```python
from build123d import *

# Parameters (mm, degrees)
SCHIZZO1_W                   = 75
SCHIZZO1_H                   = 60
ESTRUSIONE_ESTRUSIONE1_DEPTH = 5
SCHIZZO2_R                   = 5
TAGLIO_ESTRUSIONE1_DEPTH     = 49.28301979
SCHIZZO3_W                   = 45
SCHIZZO3_H                   = 5
ESTRUSIONE_ESTRUSIONE2_DEPTH = 8


with BuildPart() as part:
    # Schizzo1 → Estrusione-Estrusione1 (new body)
    with BuildSketch(Plane(origin=(0, 0, 0), x_dir=(1, 0, 0), z_dir=(0, 1, 0))):
        Rectangle(SCHIZZO1_W, SCHIZZO1_H)
    extrude(amount=ESTRUSIONE_ESTRUSIONE1_DEPTH)

    # Schizzo2 → Taglio-Estrusione1 (cut, through all)
    with BuildSketch(Plane(origin=(0, 5, 0), x_dir=(-1, 0, 0), z_dir=(0, 1, 0))):
        with Locations(Location((0, 0, 0), (0, 0, 90))):
            Circle(SCHIZZO2_R)
    extrude(amount=-TAGLIO_ESTRUSIONE1_DEPTH, mode=Mode.SUBTRACT)

    # Schizzo3 → Estrusione-Estrusione2 (add)
    with BuildSketch(Plane.XY.offset(30)):
        with Locations((0, 2.5)):
            Rectangle(SCHIZZO3_W, SCHIZZO3_H)
    estrusione_estrusione2 = extrude(amount=ESTRUSIONE_ESTRUSIONE2_DEPTH)

    # Specchia1: Estrusione-Estrusione2 across plane
    add(estrusione_estrusione2.mirror(Plane.XY))


solid = part.part
```
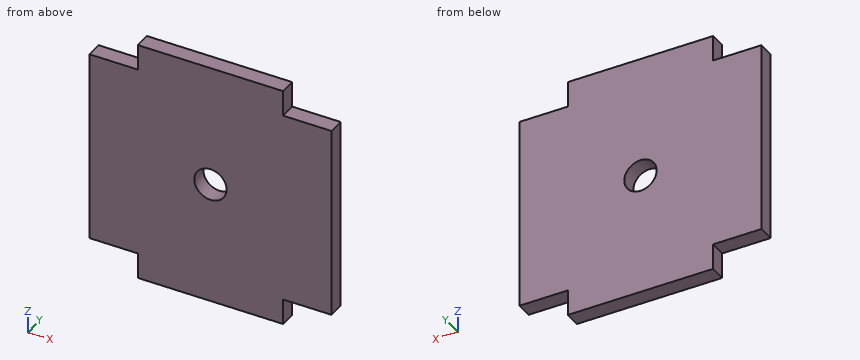
Source: CAD feature listing. Evaluate the final solid. Frame: model axes, mm. Round coordinates to 2 decimals unless told otherwise and drop trailing zeros. Order: outer loops, then holes, each group sorted by start corner. A loop starts at its lowest first (then second) coordinate and runs counter-clockwise, first axis right, second up. Notation, with made-up numbers: (88, 13.25) -> (142, 13.25) arc R20 cw to (142, 33.25) -> close; hole circle Ø4 at (48, 2.5). An arc over 180 degrees is marked (long way). Use CSV: the item, a comma, the result in double quotes.
(1) Section A-A on x = 0. Return the cut outline in (y, z), and give its area (3 significant figures).
Report:
outline,"(0, -38) -> (5, -38) -> (5, -5) -> (0, -5) -> close; (0, 5) -> (5, 5) -> (5, 38) -> (0, 38) -> close"
area,"330 mm^2"
(2) Section B-B on y = 3.25. Return the cut outline in (x, z), and give its area (3 significant figures).
Report:
outline,"(-37.5, -30) -> (-22.5, -30) -> (-22.5, -38) -> (22.5, -38) -> (22.5, -30) -> (37.5, -30) -> (37.5, 30) -> (22.5, 30) -> (22.5, 38) -> (-22.5, 38) -> (-22.5, 30) -> (-37.5, 30) -> close; hole circle Ø10 at (0, 0)"
area,"5,140 mm^2"
(3) Section D-D on x = 27.5. Return the cut outline in (y, z), and give its area (3 significant figures).
Report:
outline,"(0, -30) -> (5, -30) -> (5, 30) -> (0, 30) -> close"
area,"300 mm^2"
(4) Section C-C on z = 0. Return the cut outline in (x, y), and give its area (3 significant figures).
Report:
outline,"(-37.5, 0) -> (-5, 0) -> (-5, 5) -> (-37.5, 5) -> close; (5, 0) -> (37.5, 0) -> (37.5, 5) -> (5, 5) -> close"
area,"325 mm^2"
(5) Ray query, L1, parallel to X at y = 1.35, z = 0; L2, parallel to Z at x = -31, y = 0.7; L3, parallel to X at y = 1.95, z = -31. Return the intervals inside material, ascending.
Report:
L1,"-37.5 to -5, 5 to 37.5"
L2,"-30 to 30"
L3,"-22.5 to 22.5"
(6) First-contact query: pin 1 Ø6 at (x, z) = (-13, -28.5) entering from -Y; pin 2 Ø1.5 at (x, y) = (-31, 2.5) entering from -Z; pin 3 Ø2 at (x, z) = (-1.5, 3.5) entering from +Y; pin 4 Ø1.5 at (y, z) = (2, 35) entering from +X. Flat tips, straight axial feed; report the tip coordinate or a pass-through.
Report:
pin 1,"y = 0"
pin 2,"z = -30"
pin 3,"through"
pin 4,"x = 22.5"
